For this review, take the finished solid that the model builds, in its own axes (mm). A direction names the side the tool comes from. Round coordinates to 2 decimals unless told otherwise and drop trailing zeros. Write each loop counter-clockwise with the first axis right and the second up, starting at its lowest first coordinate (ties: lowest second). Pieces come first, ordered by that corner, then holes. Notation, with made-up numbers: M -7.75,-15.75 L 5.25,-15.75 A26 ccw 5.25,1.25 Z; hole C 76.5,54.5 d1. An arc over 180 degrees is marked long. Answer in a Markdown table with one row per item.
Autodesk Inventor part; units mm, degrees
ref_plane "Arbeitsebene1" through (0, 12, 0) normal (0, 1, 0) x (-1, 0, 0)
ref_plane "Arbeitsebene2" through (26.5, 0, 0) normal (1, 0, 0) x (0, 1, 0)
ref_plane "XY Plane" through (0, 0, 0) normal (0, 0, 1) x (1, 0, 0)
sketch "Skizze1" plane through (0, 0, 0) normal (0, 0, 1) x (1, 0, 0)
  line L0 (0, 0) -> (0, 24)
  line L1 (0, 24) -> (12, 62)
  line L2 (12, 62) -> (40, 62)
  line L3 (40, 62) -> (40, 30)
  line L4 (40, 30) -> (21, 30)
  line L5 (21, 30) -> (21, 0)
  line L6 (21, 0) -> (0, 0)
  dimension "d0" = 62
  dimension "d1" = 21
  dimension "d2" = 30
  dimension "d3" = 38
  dimension "d4" = 28
  dimension "d5" = 12
extrude "Extrusion1" add sketch "Skizze1" along normal blind 20
sketch "Skizze3" plane through (12, 62, 0) normal (0, 1, 0) x (1, 0, 0)
  line L0 (0, 0) -> (0, -20)
  line L1 (28, 0) -> (28, -20)
  point P0 (-12, 0)
  point P1 (18, -10)
  point P2 (28, -10)
  dimension "d16" = 10
hole "Bohrung2" at (30, 62, 10) direction (0, -1, 0) diameter 14 end through all
sketch "Skizze4" plane through (12, 62, 0) normal (0, 1, 0) x (1, 0, 0)
  line L0 (0, 0) -> (0, -20)
  line L1 (28, 0) -> (28, -20)
  point P0 (-12, 0)
  point P1 (4, -10)
  point P2 (28, -10)
  dimension "d24" = 4
hole "Bohrung3" at (16, 62, 10) direction (0, -1, 0) diameter 3 depth 62 counterbore diameter 4 counterbore depth 30
sketch "Skizze5" plane through (21, 0, 0) normal (1, 0, 0) x (0, 0, -1)
  line L0 (0, 0) -> (-20, 0)
  point P0 (-10, 10)
  point P1 (-10, 0)
  dimension "d32" = 10
hole "Bohrung4" at (21, 10, 10) direction (-1, 0, 0) diameter 8 depth 21 counterbore diameter 10 counterbore depth 1
ref_plane "Arbeitsebene1" through (0, 12, 0) normal (0, 1, 0) x (-1, 0, 0)
sketch "Skizze8" plane through (12, 62, 0) normal (0, 1, 0) x (1, 0, 0)
  circle A0 centre (4, -10) radius 2
  circle A1 centre (18, -10) radius 7
  line L0 (28, 0) -> (0, 0)
  line L1 (0, 0) -> (0, -20)
  line L2 (28, -20) -> (0, -20)
  line L3 (28, 0) -> (28, -20)
  line L4 (4, -10) -> (4, -3) construction
  line L5 (4, -10) -> (4, -17) construction
  line L6 (18, -10) -> (9, -10) construction
  line L7 (9, 0) -> (9, -20)
  point P0 (-12, 0)
  dimension "d57" = 14
hole "Bohrung7" at (16, 62, 17) at (16, 62, 3) direction (0, -1, 0) diameter 2.459 depth 9 tip angle 118
ref_plane "Arbeitsebene2" through (26.5, 0, 0) normal (1, 0, 0) x (0, 1, 0)
mirror "Spiegeln2" about plane through (26.5, 0, 0) normal (1, 0, 0) of "Bohrung7"
properties part number "MotorBlock" material "Glas"
Q1. Take a section at C-C (y = 57.5). State the section outline as (x, z) points, then the cut area to 3 significant figures.
Found:
| item | result |
|---|---|
| outline | M 10.58,0 L 40,0 L 40,20 L 10.58,20 Z; hole C 16,10 d4; hole C 16,3 d2.46; hole C 16,17 d2.46; hole C 30,10 d14; hole C 37,3 d2.46; hole C 37,17 d2.46 |
| area | 403 mm² |
Q2. Take a section at D-D (y = 8.5). State the section outline as (x, z) points, then the cut area to 3 significant figures.
Found:
| item | result |
|---|---|
| outline | M 0,0 L 21,0 L 21,5.23 L 20,5.23 L 20,6.29 L 0,6.29 Z; M 0,13.71 L 20,13.71 L 20,14.77 L 21,14.77 L 21,20 L 0,20 Z |
| area | 262 mm² |
Q3. Insertion check: P1, Ø3, axis at x = 16, z = 3, coming from the +Y side; P2, Ø1.8, axis at x = 16, z = 10, coming from the +Y side; P3, Ø1.2, axis at x = 15, z = 10.5, coming from the +Y side; P4, Ø2, axis at y = 36, z = 2, coming from the -X side. Each pin has a flat end and moves straight along its axis. Give the tip position at first contact, or say it passes through.
Found:
| item | result |
|---|---|
| P1 | y = 62 |
| P2 | through |
| P3 | y = 32 |
| P4 | x = 3.47 |
Q4. Take a section at A-A (z = 10). State how many separate pieces and enclosed holes the cut face has, then the cut area to 3 significant figures.
Found:
| item | result |
|---|---|
| separate pieces | 5 |
| enclosed holes | 0 |
| area | 872 mm² |
Q5. Machinability: for faces 4 (the face through (14.78, 57.44, 2.84)), 5 (the face through (36.21, 45.78, 13.23)), 6 (the face through (21, 15.2, 9.9)), which of the approach directions +Z, -Z, +X, -X, +Y, -Y give a long, thin tool a straight path to every point of the face, cutting with its end or side? Answer none if there is none.
Found:
| item | result |
|---|---|
| face 4 | +Y |
| face 5 | +Y, -Y |
| face 6 | +Z, -Z, +X, -Y |
Q6. Take a section at B-B (x = 3). State the section outline as (y, z) points, then the cut area to 3 significant figures.
Found:
| item | result |
|---|---|
| outline | M 0,0 L 33.5,0 L 33.5,20 L 0,20 Z; hole C 10,10 d8 |
| area | 620 mm² |
Q7. For probe 1 along X at (y, z) = (2.75, 10); probe 2 along Z at (x, y) = (10, 10); probe 3 along Z at (x, y) = (30, 37), list the stretches that pass through material, from the lowest coordinate up.
Found:
| item | result |
|---|---|
| probe 1 | 0 to 14.5, 17.5 to 21 |
| probe 2 | 0 to 6, 14 to 20 |
| probe 3 | 0 to 3, 17 to 20 |
Q8. Mouldability with a two-part tool opening along X and no side actions: class faces 1 (the face through (40, 46, 10)), 2 (the face through (14, 47, 10)), 3 (the face through (0, 14.5, 9.9)) as +X half, -X half, draft (parallel to the pull), parting line (faces both ways), or undercut.
Found:
| item | result |
|---|---|
| face 1 | +X half |
| face 2 | undercut |
| face 3 | -X half |
